Here's how the part is built. I have some questions about the finished solid (model axes, mm). Face numbers are marked on the shaded views. A direction names the side the tool comes from. Round coordinates to 2 decimals unless told otherwise and drop trailing zeros. Order: outer loops, then holes, each group sorted by start corner. A loop starts at its lowest first (then second) coordinate and runs counter-clockwise, first axis right, second up. Notation, with made-up numbers: (35, -4.75) - (85, -4.75) arc R21 ccw to (85, 13.25) - close; hole circle Ø6 at (-9.75, 51). An arc over 180 degrees is marked (long way). One line per item, written item: value.
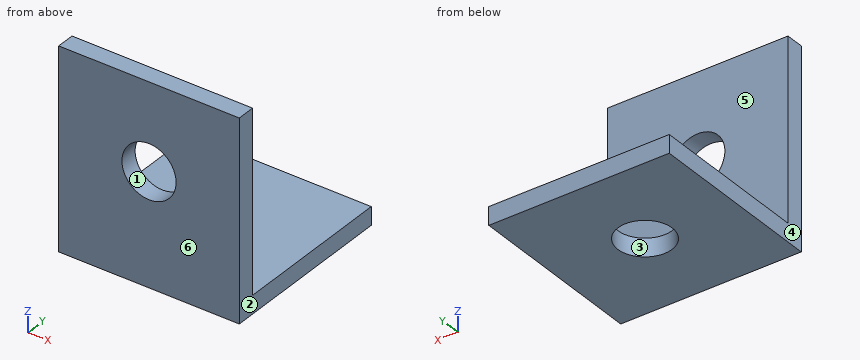
from build123d import *

# Parameters (mm, degrees)
SKETCH2_W           = 20
SKETCH2_H           = 20
BOSS_EXTRUDE1_DEPTH = 2
SKETCH3_W           = 20
SKETCH3_H           = 2
BOSS_EXTRUDE2_DEPTH = 20
SKETCH4_R           = 3
CUT_EXTRUDE1_DEPTH  = 10
SKETCH5_R           = 3
CUT_EXTRUDE2_DEPTH  = 10


with BuildPart() as part:
    # Sketch2 → Boss-Extrude1 (new body)
    with BuildSketch(Plane.XY):
        with Locations((10, 10)):
            Rectangle(SKETCH2_W, SKETCH2_H)
    extrude(amount=BOSS_EXTRUDE1_DEPTH)

    # Sketch3 → Boss-Extrude2 (add)
    with BuildSketch(Plane.XY.offset(2)):
        with Locations((10, 1)):
            Rectangle(SKETCH3_W, SKETCH3_H)
    extrude(amount=BOSS_EXTRUDE2_DEPTH)

    # Sketch4 → Cut-Extrude1 (cut)
    with BuildSketch(Plane(origin=(0, 2, 0), x_dir=(1, 0, 0), z_dir=(0, 1, 0))):
        with Locations((10, -12.415090131)):
            Circle(SKETCH4_R)
    extrude(amount=-CUT_EXTRUDE1_DEPTH, mode=Mode.SUBTRACT)

    # Sketch5 → Cut-Extrude2 (cut)
    with BuildSketch(Plane.XY.offset(2)):
        with Locations((10, 10)):
            Circle(SKETCH5_R)
    extrude(amount=-CUT_EXTRUDE2_DEPTH, mode=Mode.SUBTRACT)


solid = part.part
Q1. If we section it at A-A, the plane x = 10: Please give me the cut outline in (y, z).
Results list:
outline: (0, 0) - (7, 0) - (7, 2) - (2, 2) - (2, 9.42) - (0, 9.42) - close; (0, 15.42) - (2, 15.42) - (2, 22) - (0, 22) - close; (13, 0) - (20, 0) - (20, 2) - (13, 2) - close
Q2. If I drill on line 1 along Y through (x, z) = (10, 1.3); line 2 along Z through (x, y) = (10, 0.85); line 3 along Y through (x, z) = (13.75, 8.25), over which ranges is the centre line in solid material (lowest first)?
Results list:
line 1: 0 to 7, 13 to 20
line 2: 0 to 9.42, 15.42 to 22
line 3: 0 to 2
Q3. Which directions (+Z, -Z, +X, -X, +Y, -Y) give clear straight access to the entire face, cutting with the end or side of a thin tool? Please do the marked faces 5 and 6.
Results list:
face 5: +Z, +X, -X, +Y
face 6: +Z, -Z, +X, -X, -Y
Q4. We'd pull the mould along X, two halves only. Please class the marked faces 1, 2, 3 and 4: released by +X, released by -X, zero draft, split by the parting line, or undercut.
Results list:
face 1: undercut
face 2: released by +X
face 3: undercut
face 4: released by -X
Q5. If we section it at D-D, the plane z = 18: Please give me the cut outline in (x, y), then the cut area to 3 significant figures.
Results list:
outline: (0, 0) - (20, 0) - (20, 2) - (0, 2) - close
area: 40.0 mm²
Q6. If we section it at B-B, the plane y = 10: Please give me the cut outline in (x, z), then the cut area to 3 significant figures.
Results list:
outline: (0, 0) - (7, 0) - (7, 2) - (0, 2) - close; (13, 0) - (20, 0) - (20, 2) - (13, 2) - close
area: 28.0 mm²
Q7. Will these pins go through, and if not, where does the flat tip stop? pin 1 (9 mm diameter, centred on x = 9.5, y = 12.5, fed in from +Z); pin 2 (1.5 mm diameter, centred on x = 12.5, z = 6, fed in from +Y).
Results list:
pin 1: z = 2
pin 2: y = 2
Q8. If we section it at C-C, the plane x = 4.5: Please give me the cut outline in (y, z).
Results list:
outline: (0, 0) - (20, 0) - (20, 2) - (2, 2) - (2, 22) - (0, 22) - close
